The drawing under review shows one solid part. Ordinate dimensions are in mm from its lowest x, y, z. Coordinates: 2 decimals unless noted, no trailing zeros. Order: outer loops, then holes, each group sorted by start corner. A loop starts at its lowest first (then second) coordinate and runs counter-clockwise, first axis right, second up.
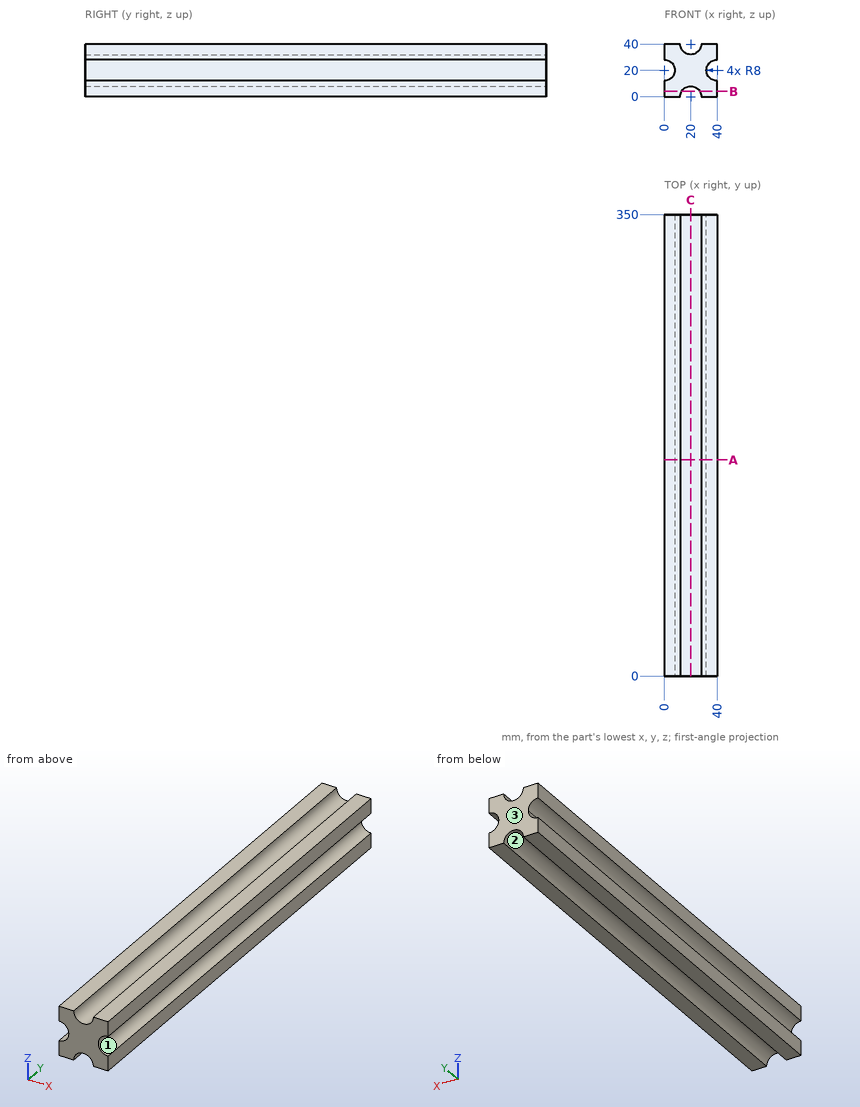
(1) We need section A-A, the plane y = 164. Write out the cut boundary in (x, z).
A:
outline: (0, 0) - (12, 0) arc R8 cw to (28, 0) - (40, 0) - (40, 12) arc R8 cw to (40, 28) - (40, 40) - (28, 40) arc R8 cw to (12, 40) - (0, 40) - (0, 28) arc R8 cw to (8, 20) arc R8 cw to (0, 12) - close
(2) Draft analysis for pull direction X (two halves, no side actions). For the marked faces 1, 2 and 3, state which applies: released by +X, released by -X, zero draft, split by the parting line, or undercut.
A:
face 1: released by +X
face 2: undercut
face 3: zero draft
(3) We need section C-C, the plane x = 20. Write out the cut boundary in (y, z), and give its area (3 significant figures).
A:
outline: (0, 8) - (350, 8) - (350, 32) - (0, 32) - close
area: 8,400 mm2
(4) Wall thickness on probe 1 along Z at (x, y) = (6.5, 144); probe 2 along X at (y, z) = (316, 33); probe 3 along X at (y, z) = (237.5, 4): over which ranges is each line inside the solid? List them lowest first.
A:
probe 1: z = 0 to 15.34, 24.66 to 40
probe 2: x = 0 to 16.13, 23.87 to 40
probe 3: x = 0 to 13.07, 26.93 to 40
(5) For pin 1 Ø1 at (x, y) = (18, 89) entering from +Z; pin 2 Ø1.5 at (y, z) = (67.5, 22.5) entering from +X, all flat-tipped, find the tip position at first contact; note any pin that passes through.
A:
pin 1: stops at z = 32.4
pin 2: stops at x = 32.69
(6) We need section B-B, the plane z = 4. Write out the cut boundary in (x, y), and give its area (3 significant figures).
A:
outline: (0, 0) - (13.07, 0) - (13.07, 350) - (0, 350) - close; (26.93, 0) - (40, 0) - (40, 350) - (26.93, 350) - close
area: 9,150 mm2
